Design review of the part built by this model. Coordinates are the model's own, in mm. A direction names the side the tool comes from. Round coordinates to 2 decimals unless told otherwise and drop trailing zeros. Loops run counter-clockwise (first coordinate to the right, second up) from the corner with the lowest first, then second, coordinate; pieces in that order, holes last. Notation, with made-up numbers: (13, 76.5) - (58, 76.5) arc R26 ccw to (58, 100.5) - close; hole circle Ø9 at (35.5, 33.25). An arc over 180 degrees is marked (long way). Return JSON: item names as keys, results as strings. Group by question number.
(1) We need section A-A, the plane y = -28. Write out the cut boundary in (x, z), and give its area (3 significant figures).
(2) Clearance check with flat-ended pins moving along their axes: pin 1 (10 mm diameter, centred on x = -34.5, y = -32, fed in from -Z); pin 2 (3.5 mm diameter, centred on x = -45.5, y = 51.73, fed in from +Z). State where each tip first meets the part, or that it passes through.
(3) Wall thickness on L1, parallel to Y at x = -41, z = 0.15; L2, parallel to Y at x = 4, z = 1.8; L3, parallel to X at y = -1, z = 1.05: over which ranges is each line inside the solid? List them lowest first. Write a range as [from, to].
(4) We need section B-B, the plane x = -18. Write out the cut boundary in (y, z).
(5) We need section D-D, the plane x = -38.5. Write out the cut boundary in (y, z).
(6) For faces 1 (the flat face through (-34, -10.273, 1)), 2 (the flat face through (-9, -46.273, 1)), list the 3-axis set-ups (+Z, -Z, +X, -X, +Y, -Y) from which the entire face can be reached by the end or side of a thin tool; tool diameter is ignored.
(7) The part is to be moulded in two halves that separate along X. For faces 3 (the flat face through (-9, 55.727, 1)), 4 (the flat face through (-34, 10.727, 1)), 5 (the flat face through (-49.498, 4, 1)), say which applies: pulls with the +X half, pulls with the -X half, needs draft (parallel to the pull), parting line crosses it, or undercut.
(8) We need section C-C, the plane z = 1.3. Write out the cut boundary in (x, y).
from build123d import *

# Parameters (mm, degrees)
SKETCH1_W                                    = 82
SKETCH1_H                                    = 102
BOSS_EXTRUDE1_DEPTH                          = 2
SKETCH2_R                                    = 9
CUT_EXTRUDE2_DEPTH                           = 2
CSK_FOR_M2_5_COUNTERSUNK_FLAT_HEAD_S_2_COUNT = 2
CSK_FOR_M2_5_COUNTERSUNK_FLAT_HEAD_S_2_PITCH = 94
CSK_FOR_M2_5_COUNTERSUNK_FLAT_HEAD_S_3_COUNT = 2
CSK_FOR_M2_5_COUNTERSUNK_FLAT_HEAD_S_3_PITCH = 119.63277143
CSK_FOR_M2_5_COUNTERSUNK_FLAT_HEAD_S_4_COUNT = 2
CSK_FOR_M2_5_COUNTERSUNK_FLAT_HEAD_S_4_PITCH = 74


with BuildPart() as part:
    # Sketch1 → Boss-Extrude1 (new body)
    with BuildSketch(Plane.XY):
        with Locations((-8.498222994, 4.726902457)):
            Rectangle(SKETCH1_W, SKETCH1_H)
    extrude(amount=BOSS_EXTRUDE1_DEPTH)

    # Sketch2 → Cut-Extrude2 (cut)
    with BuildSketch(Plane.XY.offset(2)):
        with Locations((4.301781638, 0.112195324)):
            Circle(SKETCH2_R)
        with BuildLine():
            Line((-43.498222994, -18.273097543), (26.501777006, -18.273097543))
            ThreePointArc((26.501777006, -18.273097543), (27.208883787, -18.565990762), (27.501777006, -19.273097543))
            Line((27.501777006, -19.273097543), (27.501777006, -38.273097543))
            ThreePointArc((27.501777006, -38.273097543), (27.208883787, -38.980204324), (26.501777006, -39.273097543))
            Line((26.501777006, -39.273097543), (-43.498222994, -39.273097543))
            ThreePointArc((-43.498222994, -39.273097543), (-44.205329775, -38.980204324), (-44.498222994, -38.273097543))
            Line((-44.498222994, -38.273097543), (-44.498222994, -19.273097543))
            ThreePointArc((-44.498222994, -19.273097543), (-44.205329775, -18.565990762), (-43.498222994, -18.273097543))
        make_face()
        with BuildLine():
            Line((-43.498222994, 10.726902457), (-24.498222994, 10.726902457))
            ThreePointArc((-24.498222994, 10.726902457), (-23.791116213, 10.434009238), (-23.498222994, 9.726902457))
            Line((-23.498222994, 9.726902457), (-23.498222994, -9.273097543))
            ThreePointArc((-23.498222994, -9.273097543), (-23.791116213, -9.980204324), (-24.498222994, -10.273097543))
            Line((-24.498222994, -10.273097543), (-43.498222994, -10.273097543))
            ThreePointArc((-43.498222994, -10.273097543), (-44.205329775, -9.980204324), (-44.498222994, -9.273097543))
            Line((-44.498222994, -9.273097543), (-44.498222994, 9.726902457))
            ThreePointArc((-44.498222994, 9.726902457), (-44.205329775, 10.434009238), (-43.498222994, 10.726902457))
        make_face()
    extrude(amount=-CUT_EXTRUDE2_DEPTH, mode=Mode.SUBTRACT)

    # Sketch18 → CSK for M2.5 Countersunk Flat Head Screw2 (revolve, cut)
    with BuildSketch(Plane(origin=(-45.498222994, 51.726902457, 2), x_dir=(0, -1, 0), z_dir=(1, 0, 0))):
        Polygon((0, 0), (0, 2), (1.45, 2), (1.45, 1.3), (2.75, 0), align=None)
    csk_for_m2_5_countersunk_flat_head_screw = revolve(axis=Axis((-45.498222994, 51.726902457, 8.35), (0, 0, -1)), mode=Mode.SUBTRACT)

    # CSK for M2.5 Countersunk Flat Head S 2: CSK for M2.5 Countersunk Flat Head Screw2 ×2
    with Locations(*[(0, -i * CSK_FOR_M2_5_COUNTERSUNK_FLAT_HEAD_S_2_PITCH, 0) for i in range(1, CSK_FOR_M2_5_COUNTERSUNK_FLAT_HEAD_S_2_COUNT)]):
        add(csk_for_m2_5_countersunk_flat_head_screw, mode=Mode.SUBTRACT)

    # CSK for M2.5 Countersunk Flat Head S 3: CSK for M2.5 Countersunk Flat Head Screw2 ×2
    with Locations(*[Vector(0.618559606, -0.785737878, 0) * (i * CSK_FOR_M2_5_COUNTERSUNK_FLAT_HEAD_S_3_PITCH) for i in range(1, CSK_FOR_M2_5_COUNTERSUNK_FLAT_HEAD_S_3_COUNT)]):
        add(csk_for_m2_5_countersunk_flat_head_screw, mode=Mode.SUBTRACT)

    # CSK for M2.5 Countersunk Flat Head S 4: CSK for M2.5 Countersunk Flat Head Screw2 ×2
    with Locations(*[(i * CSK_FOR_M2_5_COUNTERSUNK_FLAT_HEAD_S_4_PITCH, 0, 0) for i in range(1, CSK_FOR_M2_5_COUNTERSUNK_FLAT_HEAD_S_4_COUNT)]):
        add(csk_for_m2_5_countersunk_flat_head_screw, mode=Mode.SUBTRACT)


solid = part.part
Solutions:
{
 "1": {"outline": "(-49.5, 0) - (-44.5, 0) - (-44.5, 2) - (-49.5, 2) - close; (27.5, 0) - (32.5, 0) - (32.5, 2) - (27.5, 2) - close", "area": "20.0 mm^2"},
 "2": {"pin 1": "through", "pin 2": "z = 1"},
 "3": {"L1": "[-46.27, -39.27], [-18.27, -10.27], [10.73, 55.73]", "L2": "[-46.27, -39.27], [-18.27, -8.88], [9.11, 55.73]", "L3": "[-49.5, -44.5], [-23.5, -4.63], [13.23, 32.5]"},
 "4": {"outline": "(-46.27, 0) - (-39.27, 0) - (-39.27, 2) - (-46.27, 2) - close; (-18.27, 0) - (55.73, 0) - (55.73, 2) - (-18.27, 2) - close"},
 "5": {"outline": "(-46.27, 0) - (-39.27, 0) - (-39.27, 2) - (-46.27, 2) - close; (-18.27, 0) - (-10.27, 0) - (-10.27, 2) - (-18.27, 2) - close; (10.73, 0) - (55.73, 0) - (55.73, 2) - (10.73, 2) - close"},
 "6": {"face 1": "+Z, -Z", "face 2": "+Z, -Z, +X, -X, -Y"},
 "7": {"face 3": "needs draft", "face 4": "undercut", "face 5": "pulls with the -X half"},
 "8": {"outline": "(-49.5, -46.27) - (32.5, -46.27) - (32.5, 55.73) - (-49.5, 55.73) - close; hole circle Ø4.1 at (-45.5, -42.27); hole circle Ø4.1 at (-45.5, 51.73); hole (-44.5, -38.27) arc R1 ccw to (-43.5, -39.27) - (26.5, -39.27) arc R1 ccw to (27.5, -38.27) - (27.5, -19.27) arc R1 ccw to (26.5, -18.27) - (-43.5, -18.27) arc R1 ccw to (-44.5, -19.27) - close; hole (-44.5, -9.27) arc R1 ccw to (-43.5, -10.27) - (-24.5, -10.27) arc R1 ccw to (-23.5, -9.27) - (-23.5, 9.73) arc R1 ccw to (-24.5, 10.73) - (-43.5, 10.73) arc R1 ccw to (-44.5, 9.73) - close; hole circle Ø18 at (4.3, 0.11); hole circle Ø4.1 at (28.5, -42.27); hole circle Ø4.1 at (28.5, 51.73)"}
}
